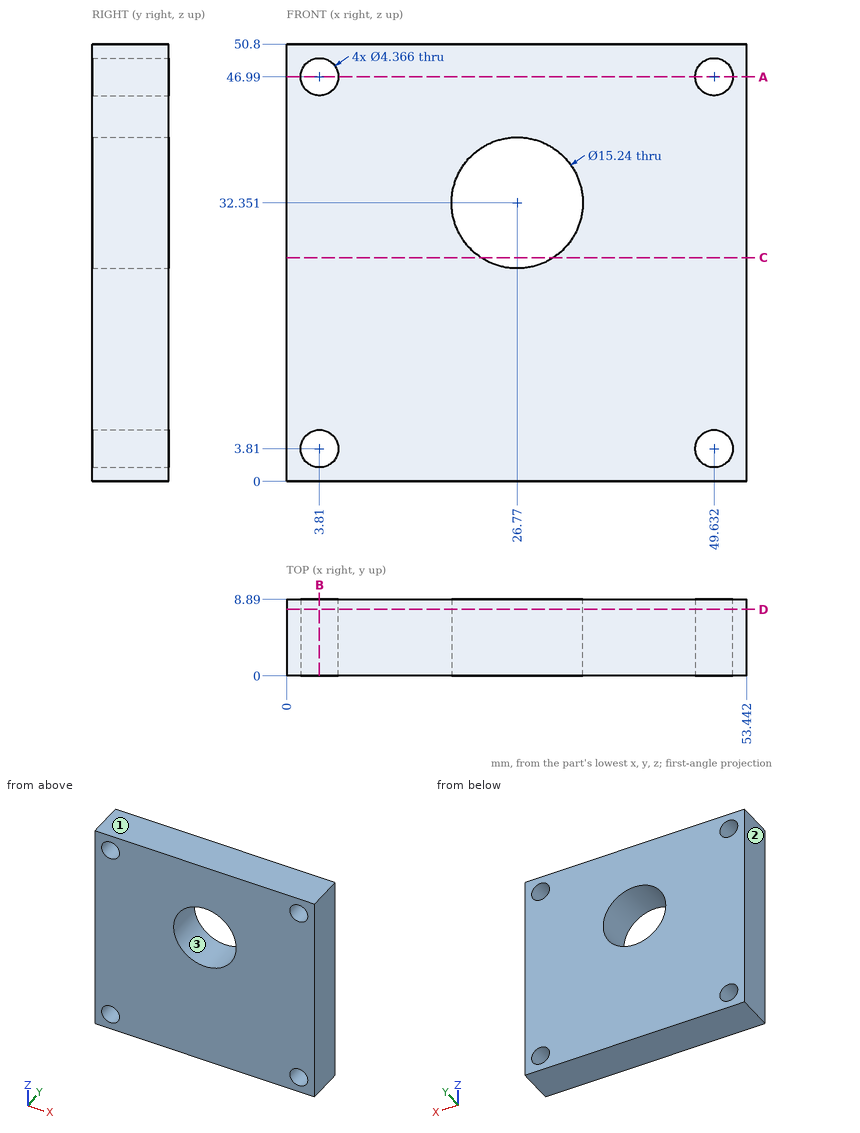
Design review of the part shown in the three views and the two pictorial views. Dimensions are in mm from the part's minimum x, y and z. Give positions to 0.01 mm unless a question says otherwise; leave off trailing zeros. Loops run counter-clockwise (first coordinate to the right, second up) from the corner with the lowest first, then second, coordinate; pieces in that order, holes last. Notation, with made-up numbers: M 30,7 L 44,7 A21 cw 44,30 Z; hole C 7.5,-19 d11. An arc over 180 degrees is marked long. Answer as a JSON object with one key per item and string values. Group by question number.
Q1. Add section B-B on x = 3.81. Give the boundary of the cut face in (y, z), and give its area (3 significant figures).
Q2. Add section D-D on y = 7.75. Give the number of separate pieces and of enclosed holes in the cut face, and give its area (3 significant figures).
Q3. Mouldability with a two-part tool opening along Z and no side actions: class the marked faces 1, 2 and 3 as +Z half, -Z half, draft (parallel to the pull), parting line (faces both ways), or undercut.
Q4. Add section A-A on z = 46.99. Give the boundary of the cut face in (x, y) (1 decimal).
Q5. Add section C-C on z = 26. Give the boundary of the cut face in (x, y), and give its area (3 significant figures).
Q6. Insertion check: P1, Ø24.5, axis at x = 26.77, z = 32.35, coming from the +Y side; P2, Ø2.5, axis at x = 3.81, z = 46.99, coming from the +Y side. Each pin has a flat end and moves straight along its axis. Give the tip position at first contact, or say it passes through.
Q7. For probe 1 along X at (y, z) = (3.5, 47) (1 decimal); probe 2 along X at (y, z) = (5, 4) (1 decimal); probe 3 along Z at (x, y) = (3.81, 4), list the stretches that pass through material, from the lowest coordinate up. Write a range as [from, to].
Checked values:
{
 "1": {"outline": "M 0,0 L 8.89,0 L 8.89,1.63 L 0,1.63 Z; M 0,5.99 L 8.89,5.99 L 8.89,44.81 L 0,44.81 Z; M 0,49.17 L 8.89,49.17 L 8.89,50.8 L 0,50.8 Z", "area": "374 mm²"},
 "2": {"separate pieces": "1", "enclosed holes": "5", "area": "2,470 mm²"},
 "3": {"face 1": "+Z half", "face 2": "draft", "face 3": "undercut"},
 "4": {"outline": "M 0,0 L 1.6,0 L 1.6,8.9 L 0,8.9 Z; M 6,0 L 47.4,0 L 47.4,8.9 L 6,8.9 Z; M 51.8,0 L 53.4,0 L 53.4,8.9 L 51.8,8.9 Z"},
 "5": {"outline": "M 0,0 L 22.56,0 L 22.56,8.89 L 0,8.89 Z; M 30.98,0 L 53.44,0 L 53.44,8.89 L 30.98,8.89 Z", "area": "400 mm²"},
 "6": {"P1": "y = 8.89", "P2": "through"},
 "7": {"probe 1": "[0, 1.6], [6, 47.4], [51.8, 53.4]", "probe 2": "[0, 1.6], [6, 47.5], [51.8, 53.4]", "probe 3": "[0, 1.63], [5.99, 44.81], [49.17, 50.8]"}
}
